Design review of the part built by this model. Coordinates are the model's own, in mm. Give positions to 0.01 mm unless a question says otherwise; leave off trailing zeros. Loops run counter-clockwise (first coordinate to the right, second up) from the corner with the lowest first, then second, coordinate; pieces in that order, holes last.
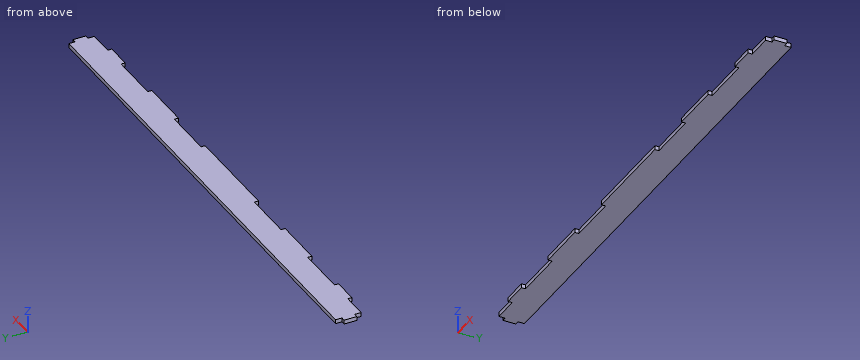
from build123d import *

# Parameters (mm, degrees)
F0_W     = 10
F0_H     = 1.5875
F0_W_2   = 1.5875
F0_H_2   = 5
F0_W_3   = 20
F0_W_4   = 40
F1_DEPTH = 1.5875


# Not quite as in the source:
# - a length typed as a fraction of an inch, garbled in the dataset ("3 / 203.2 mm" for 3/8 in), is restored


with BuildPart() as f1:
    # F0 (on Top) → F1 (new body)
    with BuildSketch(Plane.XY):
        Polygon((-100, -2.5), (-100, -5), (-90, -5), (-80, -5), (-60, -5), (-40, -5), (-20, -5), (20, -5), (40, -5), (60, -5), (80, -5), (90, -5), (100, -5), (100, -2.5), (100, 2.5), (100, 5), (-100, 5), (-100, 2.5), align=None)
        with Locations((-85, -5.79375)):
            Rectangle(F0_W, F0_H)
        with Locations((-100.79375, 0)):
            Rectangle(F0_W_2, F0_H_2)
        with Locations((-50, -5.79375)):
            Rectangle(F0_W_3, F0_H)
        with Locations((0, -5.79375)):
            Rectangle(F0_W_4, F0_H)
        with Locations((100.79375, 0)):
            Rectangle(F0_W_2, F0_H_2)
        with Locations((50, -5.79375)):
            Rectangle(F0_W_3, F0_H)
        with Locations((85, -5.79375)):
            Rectangle(F0_W, F0_H)
    extrude(amount=F1_DEPTH)


solid = f1.part
Q1. Take a section at B-B (x = 71). Give the boundary of the cut face in (y, z), plus the area to 3 significant figures.
Results:
outline: (-5, 0) - (5, 0) - (5, 1.59) - (-5, 1.59) - close
area: 15.9 mm2
Q2. Wall thickness on line 1 (X direction, y = -5.75, z = 0.7); line 2 (X direction, y = -4, z = 0.8); line 3 (Y direction, x = 28, z = 0.65): over which ranges is each line inside the solid? List them lowest first.
Results:
line 1: x = -90 to -80, -60 to -40, -20 to 20, 40 to 60, 80 to 90
line 2: x = -100 to 100
line 3: y = -5 to 5
Q3. Insertion check: pin 1 (0.8 mm diameter, centred on x = -67, z = 1, fed in from -Y); pin 2 (0.5 mm diameter, centred on y = -6, z = 0.5, fed in from -X); pin 3 (0.8 mm diameter, centred on x = -101, z = 1, fed in from -Y). Each pin has a flat end and moves straight along its axis. Give the tip position at first contact, or say it passes through.
Results:
pin 1: stops at y = -5
pin 2: stops at x = -90
pin 3: stops at y = -2.5
